The listing builds one solid part. Answer for the finished solid, in the listing's coordinates (mm). Face numbers are marked on the shaded views. A direction names the side the tool comes from. Round coordinates to 2 decimals unless told otherwise and drop trailing zeros. Loops run counter-clockwise (first coordinate to the right, second up) from the corner with the lowest first, then second, coordinate; pieces in that order, holes last. Notation, with made-up numbers: (-5.5, 56) -> (1.5, 56) arc R29 ccw to (1.5, 93) -> close; hole circle Ø1 at (-2.5, 68.5). An arc over 180 degrees is marked (long way). Use a Markdown table: item, result. Add a question column.
Q1. Section B-B on x = -6 is taken. Give the vertices of the cut face in (y, z).
Q2. Which of the six approach directions +Z, -Z, +X, -X, +Y, -Y give full straight-line access (tool end or side, diameter ignored) to the marked faces 4 and 5?
Q3. Section D-D on x = 1 is taken. Give the vertices of the cut face in (y, z), then the cut area to 3 significant figures.
Q4. Section A-A on z = -7 is taken. Give the vertices of the cut face in (x, y).
Q5. Section C-C on z = 7 is taken. Give the vertices of the cut face in (x, y).
Q6. For a pull along X with two mould halves and no side action, classify the marked faces 1, 2 and 3 as released by +X, released by -X, zero draft, split by the parting line, or undercut.
Q7. Consider line 1 (X direction, y = 0.75, z = 7); line 2 (X direction, y = 2.2, z = -2.5); line 3 (X direction, y = 1.05, z = -7). Determine where each line is inside the solid, lowest interval first.
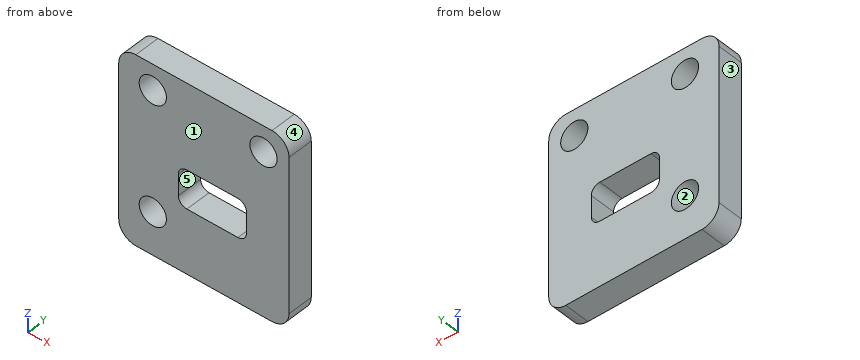
from build123d import *

# Parameters (mm, degrees)
SKETCH_2_W      = 20
SKETCH_2_H      = 22
SKETCH_2_R      = 1.6
SKETCH_2_W_2    = 8
SKETCH_2_H_2    = 4.5
EXTRUDE_1_DEPTH = 3
FILLET_1_R      = 2
FILLET_2_R      = 1


with BuildPart() as part:
    # 草图2 → 凸台-拉伸1 (new body)
    with BuildSketch(Plane(origin=(0, 0, 0), x_dir=(1, 0, 0), z_dir=(0, 1, 0))):
        with Locations((0, 1)):
            Rectangle(SKETCH_2_W, SKETCH_2_H)
        with Locations(Location((-6, -7, 0), (0, 0, 270))):
            Circle(SKETCH_2_R, mode=Mode.SUBTRACT)
        with Locations(Location((7, -7, 0), (0, 0, 270))):
            Circle(SKETCH_2_R, mode=Mode.SUBTRACT)
        with Locations(Location((-6, 7, 0), (0, 0, 270))):
            Circle(SKETCH_2_R, mode=Mode.SUBTRACT)
        with Locations((1, 2.25)):
            Rectangle(SKETCH_2_W_2, SKETCH_2_H_2, mode=Mode.SUBTRACT)
    extrude(amount=EXTRUDE_1_DEPTH)

    # 圆角1
    fillet_1_edges = [part.edges().sort_by_distance(p)[0] for p in [
        (10, 1.5, 10),
        (-10, 1.5, 10),
        (-10, 1.5, -12),
        (10, 1.5, -12),
    ]]
    fillet(fillet_1_edges, radius=FILLET_1_R)

    # 圆角2
    fillet_2_edges = [part.edges().sort_by_distance(p)[0] for p in [
        (5, 1.5, -4.5),
        (-3, 1.5, -4.5),
        (-3, 1.5, 0),
        (5, 1.5, 0),
    ]]
    fillet(fillet_2_edges, radius=FILLET_2_R)


solid = part.part
Checked values:
| question | item | result |
|---|---|---|
| 1 | outline | (0, -12) -> (3, -12) -> (3, -8.6) -> (0, -8.6) -> close; (0, -5.4) -> (3, -5.4) -> (3, 5.4) -> (0, 5.4) -> close; (0, 8.6) -> (3, 8.6) -> (3, 10) -> (0, 10) -> close |
| 2 | face 4 | +Z, +X, +Y, -Y |
| 2 | face 5 | +Y, -Y |
| 3 | outline | (0, -12) -> (3, -12) -> (3, -4.5) -> (0, -4.5) -> close; (0, 0) -> (3, 0) -> (3, 10) -> (0, 10) -> close |
| 3 | area | 52.5 mm2 |
| 4 | outline | (-10, 0) -> (-7.6, 0) -> (-7.6, 3) -> (-10, 3) -> close; (-4.4, 0) -> (10, 0) -> (10, 3) -> (-4.4, 3) -> close |
| 5 | outline | (-10, 0) -> (-7.6, 0) -> (-7.6, 3) -> (-10, 3) -> close; (-4.4, 0) -> (5.4, 0) -> (5.4, 3) -> (-4.4, 3) -> close; (8.6, 0) -> (10, 0) -> (10, 3) -> (8.6, 3) -> close |
| 6 | face 1 | zero draft |
| 6 | face 2 | undercut |
| 6 | face 3 | released by -X |
| 7 | line 1 | x = -10 to -7.6, -4.4 to 5.4, 8.6 to 10 |
| 7 | line 2 | x = -10 to -3, 5 to 10 |
| 7 | line 3 | x = -10 to -7.6, -4.4 to 10 |
